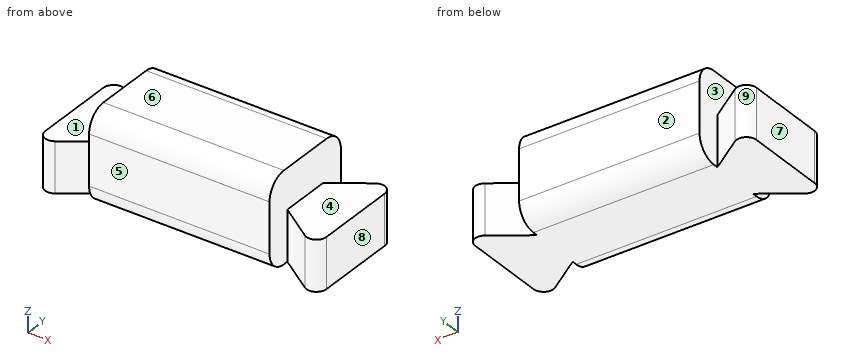
from build123d import *

# Parameters (mm, degrees)
F1_DEPTH = 9
F2_R     = 2
F3_DEPTH = 5
F4_R     = 1


with BuildPart() as f1:
    # F0 (on Top) → F1 (new body)
    with BuildSketch(Plane.XY):
        Polygon((9, 5), (0, 5), (-9, 5), (-9, 2.5), (-9, -2.5), (-9, -5), (0, -5), (9, -5), (9, -2.5), (9, 0), (9, 2.5), align=None)
    extrude(amount=F1_DEPTH)

    # F2
    f2_edges = [f1.edges().sort_by_distance(p)[0] for p in [
        (0, -5, 9),
        (0, 5, 9),
        (0, 5, 0),
        (0, -5, 0),
    ]]
    fillet(f2_edges, radius=F2_R)

    # F0 (on Top) → F3 (join)
    with BuildSketch(Plane.XY):
        Polygon((14.0249378106, 6), (9, 2.5), (9, 0), (14.0249378106, 0), align=None)
        Polygon((14.0249378106, 0), (9, 0), (9, -2.5), (14.0249378106, -6), align=None)
        Polygon((-9, -2.5), (-9, 2.5), (-14.0249378106, 6), (-14.0249378106, -6), align=None)
    extrude(amount=F3_DEPTH)

    # F4
    f4_edges = [f1.edges().sort_by_distance(p)[0] for p in [
        (-14.024938, 6, 2.5),
        (-14.024938, -6, 2.5),
        (14.024938, -6, 2.5),
        (14.024938, 6, 2.5),
    ]]
    fillet(f4_edges, radius=F4_R)


solid = f1.part
Model file for the job. Use its own axes, mm. Face numbers are marked on the shaded views. A direction names the side the tool comes from. Give positions to 0.01 mm unless a question says otherwise; leave off trailing zeros. Write each loop counter-clockwise with the first axis right and the second up, starting at its lowest first coordinate (ties: lowest second). Pieces come first, ordered by that corner, then holes. Notation, with made-up numbers: (-37.75, 14) -> (-24.75, 14) arc R12 ccw to (-24.75, 31) -> close; hole circle Ø11 at (67, 87). An arc over 180 degrees is marked (long way). Write item = value, one per line.
(1) Probe line 1 along X through (y, z) = (4.5, 2.5); line 2 along Z through (x, y) = (-12.25, 2); line 3 along X through (y, z) = (2.75, 7.25). List the from-to ranges inside material, lowest first.
Determined:
line_1 = -13.93 to -11.87, -9 to 9, 11.87 to 13.93
line_2 = 0 to 5
line_3 = -9 to 9
(2) Tool access for the marked faces 1, 2, 3, 4 and 5: list every direction of +Z, -Z, +X, -X, +Y, -Y with a clear straight run to the whole face (end or side of a thin tool).
Determined:
face_1 = +Z, -X, +Y, -Y
face_2 = +Z, -Z, +Y
face_3 = +Z
face_4 = +Z, +X, +Y, -Y
face_5 = +Z, -Z, -Y
(3) Slice it at A-A, the plane y = -3.5. Give the cut face in (x, z), then the cut area to 3 significant figures.
Determined:
outline = (-14.02, 0) -> (-10.44, 0) -> (-10.44, 5) -> (-14.02, 5) -> close; (-9, 0.06) -> (9, 0.06) -> (9, 8.94) -> (-9, 8.94) -> close; (10.44, 0) -> (14.02, 0) -> (14.02, 5) -> (10.44, 5) -> close
area = 196 mm2
(4) Slice it at D-D, the plane z = 6.5. Give the cut face in (x, y).
Determined:
outline = (-9, -5) -> (9, -5) -> (9, 5) -> (-9, 5) -> close
(5) Slice it at C-C, the plane y = 2. Give the cut face in (x, z), then the cut area to 3 significant figures.
Determined:
outline = (-14.02, 0) -> (14.02, 0) -> (14.02, 5) -> (9, 5) -> (9, 9) -> (-9, 9) -> (-9, 5) -> (-14.02, 5) -> close
area = 212 mm2
(6) Slice it at B-B, the plane x = 3.25. Give the cut face in (y, z), then the cut area to 3 significant figures.
Determined:
outline = (-5, 2) arc R2 ccw to (-3, 0) -> (3, 0) arc R2 ccw to (5, 2) -> (5, 7) arc R2 ccw to (3, 9) -> (-3, 9) arc R2 ccw to (-5, 7) -> close
area = 86.6 mm2
(7) Mould opens along X. For the marked faces 6, 7, 8 and 9 say: released by +X, released by -X, zero draft, split by the parting line, or undercut.
Determined:
face_6 = zero draft
face_7 = released by -X
face_8 = released by +X
face_9 = undercut
(8) Flat gauge pins, fed straight in: P1, Ø4.5, axis at y = -1.5, z = 6.5, coming from the -X side; P2, Ø1.5, axis at x = 11.5, y = -2, coming from the +Z side; P3, Ø2.5, axis at x = 4, z = 3.5, coming from the +Y side; P4, Ø4, axis at x = 3, z = 4.5, coming from the -Y side. Where does each tip first touch, or does it go through?
Determined:
P1 = -14.02
P2 = 5
P3 = 5
P4 = -5
